Geometry: final body of the model. Coordinates: model frame, mm. Face numbers are marked on the shaded views. A direction names the side the tool comes from. Give positions to 0.01 mm unless a question says otherwise; leave off trailing zeros. Loops run counter-clockwise (first coordinate to the right, second up) from the corner with the lowest first, then second, coordinate; pieces in that order, holes last. Notation, with made-up numbers: (39, 62.5) -> (53, 62.5) arc R15 ccw to (53, 86.5) -> close; hole circle Ø1 at (41.5, 82.25). An arc over 180 degrees is marked (long way). Answer in a Markdown table with one row per item. Add a question column.
from build123d import *

# Parameters (mm, degrees)
F1_DEPTH = 63.5
F0_W     = 25.5854227781
F0_H     = 19.05
F2_DEPTH = 25.4
F3_DEPTH = 7.9375
F5_R     = 6.35


# Not quite as in the source:
# - a feature names something its author has since deleted; it is built from what else it names


with BuildPart() as f1:
    # F0 (on Front) → F1 (new body, symmetric)
    with BuildSketch(Plane.XZ):
        Polygon((22.225, 4.044502968), (-41.275, 4.044502968), (-41.275, -15.005497032), (41.275, -15.005497032), (41.275, 4.044502968), align=None)
    extrude(amount=F1_DEPTH, both=True)

    # F0 (on Front) → F2 (join, symmetric)
    with BuildSketch(Plane.XZ):
        with BuildLine():
            Line((22.225, 21.519702968), (22.225, 4.044502968))
            Line((22.225, 4.044502968), (41.275, 4.044502968))
            Line((41.275, 4.044502968), (41.275, 21.519702968))
            ThreePointArc((41.275, 21.519702968), (45.9246798487, 32.7450231193), (57.15, 37.394702968))
            Line((57.15, 37.394702968), (60.1395772219, 37.394702968))
            Line((60.1395772219, 37.394702968), (60.1395772219, 56.444702968))
            Line((60.1395772219, 56.444702968), (57.15, 56.444702968))
            ThreePointArc((57.15, 56.444702968), (32.4542956671, 46.2154073009), (22.225, 21.519702968))
        make_face()
        with Locations((72.9322886109, 46.919702968)):
            Rectangle(F0_W, F0_H)
    extrude(amount=F2_DEPTH, both=True)

    # F0 (on Front) → F3 (join, symmetric)
    with BuildSketch(Plane.XZ):
        with BuildLine():
            add(Edge.make_bspline(
                [(-41.275, 4.044502968), (-41.275, 26.4462009072), (13.2231097668, 56.444702968), (57.15, 56.444702968)],
                knots=[0, 0, 0, 0, 111.5045361635, 111.5045361635, 111.5045361635, 111.5045361635], degree=3))
            Line((-41.275, 4.044502968), (22.225, 4.044502968))
            Line((22.225, 4.044502968), (22.225, 21.519702968))
            ThreePointArc((22.225, 21.519702968), (32.4542956671, 46.2154073009), (57.15, 56.444702968))
        make_face()
    extrude(amount=F3_DEPTH, both=True)

    # F0 (on Front) → F4 (revolve)
    with BuildSketch(Plane.XZ):
        Polygon((85.725, 61.194502968), (85.725, 56.444702968), (85.725, 37.394702968), (85.725, 32.619502968), (110.9395772219, 32.619502968), (110.9395772219, 61.194502968), align=None)
    revolve(axis=Axis((85.725, 0, 46.907002968), (0, 0, -1)))

    # F5
    f5_edges = [f1.edges().sort_by_distance(p)[0] for p in [
        (-41.275, -63.5, -5.480497),
        (41.275, -63.5, -5.480497),
        (41.275, 63.5, -5.480497),
        (-41.275, 63.5, -5.480497),
    ]]
    fillet(f5_edges, radius=F5_R)


solid = f1.part
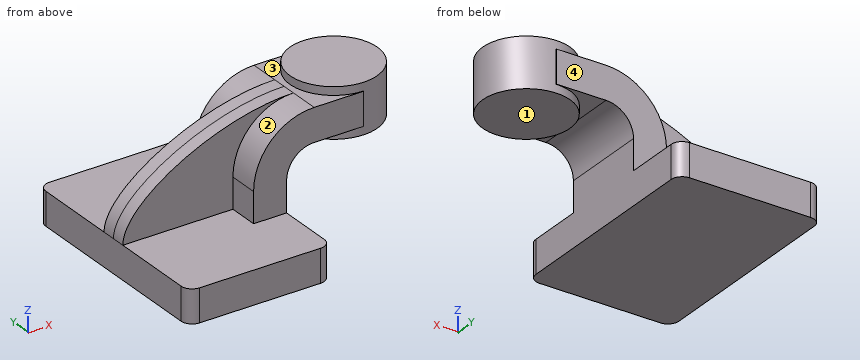
(1) Reachability of the marked faces 1, 2, 3 and 4 from +Z, -Z, +X, -X, +Y, -Y: full face, straight path, thin tool, end or side. Return the list, or none.
(2) Pin query (flat end, axial travel): pin 1 Ø8 at (x, z) = (40, -0.5) entering from +Y; pin 2 Ø12 at (x, y) = (-5, -30.5) entering from +Z; pin 3 Ø3 at (x, z) = (6, 13.5) entering from -Y. Return the tip coordinate at first contact, or that it passes through.
(3) Cut plane B-B on y = -48. Return the cut outline in (x, z) (1 decimal), then the cut area to 3 significant figures.
(4) Material intervals for line 1 along Z through (x, y) = (97, -2); line 2 along Z through (x, y) = (-1.5, 11.5); line 3 along X through (y, z) = (-54, 3.5) (3 decimals), sorted ascending. Write a range as from..to.
Answer list:
| question | item | result |
|---|---|---|
| 1 | face 1 | -Z, +X, +Y, -Y |
| 1 | face 2 | +Z, -X, -Y |
| 1 | face 3 | +Z, -X |
| 1 | face 4 | +Z, +X, -X, +Y |
| 2 | pin 1 | stops at y = 63.41 |
| 2 | pin 2 | stops at z = 4.04 |
| 2 | pin 3 | stops at y = -7.94 |
| 3 | outline | (-41.3, -15) -> (41.3, -15) -> (41.3, 4) -> (-41.3, 4) -> close |
| 3 | area | 1,570 mm² |
| 4 | line 1 | z = 32.62..61.19 |
| 4 | line 2 | z = -15.01..4.04 |
| 4 | line 3 | x = -41.275..41.275 |
